Check sheet for the modelled part. Datum: model origin and axes. Units: mm. Face numbers are marked on the shaded views. A direction names the side the tool comes from. Round coordinates to 2 decimals unless told otherwise and drop trailing zeros. Order: outer loops, then holes, each group sorted by start corner. A loop starts at its lowest first (then second) coordinate and runs counter-clockwise, first axis right, second up. Notation, with made-up numbers: (-30, 38.25) -> (-22, 38.25) arc R28 ccw to (-22, 59.25) -> close; hole circle Ø2 at (21, -18.5). An arc over 180 degrees is marked (long way). Use CSV: the item, a comma, the result in double quotes.
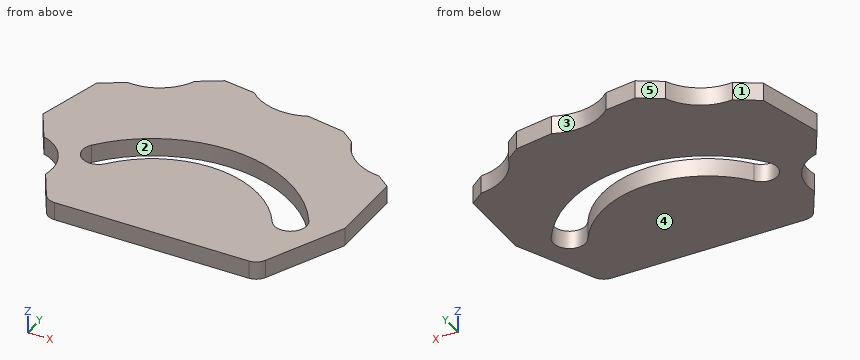
```python
from build123d import *

# Parameters (mm, degrees)
BOSS_EXTRUDE1_DEPTH = 4
FILLET1_R           = 3


with BuildPart() as part:
    # Sketch1 → Boss-Extrude1 (new body)
    with BuildSketch(Plane.XY):
        with BuildLine():
            Line((-146.758239428, -31.610515221), (-100.258239428, -31.610515221))
            Line((-100.258239428, -31.610515221), (-91.398393923, -12.610515221))
            Line((-91.398393923, -12.610515221), (-91.398393923, 4.389484779))
            Line((-91.398393923, 4.389484779), (-94.509492228, 6.780828765))
            ThreePointArc((-94.509492228, 6.780828765), (-100.889202751, 9.230316509), (-104.897213893, 14.765345257))
            Line((-104.897213893, 14.765345257), (-108.065854757, 17.200919299))
            Line((-108.065854757, 17.200919299), (-116.565854757, 18.652315204))
            ThreePointArc((-116.565854757, 18.652315204), (-123.504827753, 17.774994873), (-129.759511963, 20.90516462))
            Line((-129.759511963, 20.90516462), (-136.759511963, 21.888950463))
            Line((-136.759511963, 21.888950463), (-141.759511963, 18.884647367))
            ThreePointArc((-141.759511963, 18.884647367), (-146.29133737, 13.762936165), (-152.973799535, 12.308953164))
            Line((-152.973799535, 12.308953164), (-158.116803339, 9.218724715))
            Line((-158.116803339, 9.218724715), (-161.999089016, -5.27016268))
            Line((-161.999089016, -5.27016268), (-157.957637132, -12.27016268))
            ThreePointArc((-157.957637132, -12.27016268), (-152.397461521, -16.623171082), (-151.377041582, -23.610515221))
            Line((-151.377041582, -23.610515221), (-146.758239428, -31.610515221))
        make_face()
        with BuildLine():
            ThreePointArc((-98.776012151, -13.587867208), (-122.779946794, 0.93416519), (-148.448407118, -10.388751744))
            ThreePointArc((-148.448407118, -10.388751744), (-147.89790448, -15.381816967), (-142.904839257, -14.83131433))
            ThreePointArc((-142.904839257, -14.83131433), (-123.236532063, -6.155195631), (-104.843657911, -17.282617793))
            ThreePointArc((-104.843657911, -17.282617793), (-99.962459738, -18.46906538), (-98.776012151, -13.587867208))
        make_face(mode=Mode.SUBTRACT)
    extrude(amount=BOSS_EXTRUDE1_DEPTH)

    # Fillet1
    fillet1_edges = [part.edges().sort_by_distance(p)[0] for p in [
        (-146.758239428, -31.610515221, 2),
        (-100.258239428, -31.610515221, 2),
    ]]
    fillet(fillet1_edges, radius=FILLET1_R)


solid = part.part
```
Q1. Sectioned sample at B-B, the plane x = -125.5. Enter the section's corners in (y, z).
Result sheet:
outline,"(-31.61, 0) -> (-6.12, 0) -> (-6.12, 4) -> (-31.61, 4) -> close; (0.99, 0) -> (18.29, 0) -> (18.29, 4) -> (0.99, 4) -> close"
Q2. Mould release check, pull along X, two halves, no side actions. Record for the marked faces 3, 4 and 5: pulls with the +X half, pulls with the -X half, needs draft (parallel to the pull), parting line crosses it, or undercut.
Result sheet:
face 3,"undercut"
face 4,"needs draft"
face 5,"pulls with the -X half"
Q3. Access from +Z, -Z, +X, -X, +Y, -Y to the whole of each face (thin tool, end or side, straight path). Record for the marked faces 1 and 2.
Result sheet:
face 1,"+Z, -Z, -X, +Y"
face 2,"+Z, -Z"
Q4. Sectioned sample at C-C, the plane z = 2.4. Enter the section's corners in (x, y), then the cut area to 3 significant figures.
Result sheet:
outline,"(-162, -5.27) -> (-157.96, -12.27) arc R9.5 cw to (-151.38, -23.61) -> (-147.62, -30.11) arc R3 ccw to (-145.03, -31.61) -> (-102.17, -31.61) arc R3 ccw to (-99.45, -29.88) -> (-91.4, -12.61) -> (-91.4, 4.39) -> (-94.51, 6.78) arc R12 cw to (-104.9, 14.77) -> (-108.07, 17.2) -> (-116.57, 18.65) arc R12.03 cw to (-129.76, 20.91) -> (-136.76, 21.89) -> (-141.76, 18.88) arc R11 cw to (-152.97, 12.31) -> (-158.12, 9.22) -> close; hole (-148.45, -10.39) arc R3.55 ccw to (-142.9, -14.83) arc R23.29 cw to (-104.84, -17.28) arc R3.55 ccw to (-98.78, -13.59) arc R30.39 ccw to start"
area,"2,540 mm^2"
Q5. Sectioned sample at A-A, the plane y = -0.5. Enter the section's corners in (x, z), then the cut area to 3 significant figures.
Result sheet:
outline,"(-160.72, 0) -> (-134.15, 0) -> (-134.15, 4) -> (-160.72, 4) -> close; (-115.31, 0) -> (-91.4, 0) -> (-91.4, 4) -> (-115.31, 4) -> close"
area,"202 mm^2"
Q6. Go/stop test with a flat-tipped pin: pin 1 (2 mm diameter, centred on y = 13, z = 3.5, fed in from +X). Record where the tip stops, or that it passes through.
Result sheet:
pin 1,"stops at x = -103.5"
Q7. Scan lines: L1, parallel to X at y = -11, z = 3.35; L2, parallel to Y at x = -137.5, z = 3.4; L3, parallel to Y at x = -146.5, z = 3.55. Record each from-to range of solid material in increasing order.
Result sheet:
L1,"x = -158.69 to -148.84, -139.01 to -110.45, -100.54 to -91.4"
L2,"y = -31.61 to -9.92, -1.81 to 21.44"
L3,"y = -31.22 to -16.07, -8.19 to 13.64"
